from build123d import *

# Parameters (mm, degrees)
SKETCH2_W           = 635
SKETCH2_H           = 635
BOSS_EXTRUDE3_DEPTH = 4.445
SKETCH3_R           = 3.175
SKETCH3_R_2         = 3.9751
CUT_EXTRUDE1_DEPTH  = 631.349772348
SKETCH4_W           = 635
SKETCH4_H           = 635
SKETCH4_R           = 3.175
CUT_EXTRUDE2_DEPTH  = 631.349772348


with BuildPart() as part:
    # Sketch2 → Boss-Extrude3 (new body)
    with BuildSketch(Plane.XY):
        with Locations((164.767692446, -88.380463065)):
            Rectangle(SKETCH2_W, SKETCH2_H)
    extrude(amount=BOSS_EXTRUDE3_DEPTH)

    # Sketch3 → Cut-Extrude1 (cut, through all)
    with BuildSketch(Plane(origin=(0, 0, 0), x_dir=(-1, 0, 0), z_dir=(0, 0, -1))):
        with Locations((-138.143199548, 71.871365193)):
            Circle(SKETCH3_R)
        with Locations((-198.809547248, -25.000118004)):
            Circle(SKETCH3_R)
        with Locations((-122.004659563, -96.265887155)):
            Circle(SKETCH3_R)
        with Locations((-26.754659563, 23.469712845)):
            Circle(SKETCH3_R_2)
    extrude(amount=-CUT_EXTRUDE1_DEPTH, mode=Mode.SUBTRACT)

    # Sketch4 → Cut-Extrude2 (cut, through all)
    # profile 1 of 9: a face of its own
    with BuildSketch(Plane.XY.offset(4.445)):
        with Locations((164.767692446, -88.380463065)):
            Rectangle(SKETCH4_W, SKETCH4_H)
        with BuildLine():
            Line((-77.2226341, -77.634727654), (8.633248965, 17.594597704))
            ThreePointArc((8.633248965, 17.594597704), (15.63151489, 38.935098471), (38.089671454, 38.780493538))
            Line((38.089671454, 38.780493538), (119.216168571, 74.032383096))
            ThreePointArc((119.216168571, 74.032383096), (143.785411305, 90.066637834), (154.972256192, 62.944699943))
            Line((154.972256192, 62.944699943), (198.125737804, -5.962394804))
            ThreePointArc((198.125737804, -5.962394804), (212.645203515, -11.905190907), (217.780898828, -26.729371954))
            Line((217.780898828, -26.729371954), (291.816561623, -78.971587768))
            ThreePointArc((291.816561623, -78.971587768), (317.962531349, -102.027327271), (283.306875621, -105.790887155))
            Line((283.306875621, -105.790887155), (138.502443505, -105.790887155))
            ThreePointArc((138.502443505, -105.790887155), (122.004659563, -115.315887155), (105.506875621, -105.790887155))
            Line((105.506875621, -105.790887155), (-64.697556495, -105.790887155))
            ThreePointArc((-64.697556495, -105.790887155), (-98.60087325, -104.008621005), (-77.2226341, -77.634727654))
        make_face(mode=Mode.SUBTRACT)
    # profile 2 of 9: a face of its own
    with BuildSketch(Plane.XY.offset(4.445)):
        with BuildLine():
            Line((146.273652248, -86.740887155), (269.785475941, -86.740887155))
            Line((269.785475941, -86.740887155), (206.797645188, -42.294417391))
            ThreePointArc((206.797645188, -42.294417391), (200.080272342, -44.007689067), (193.194620104, -43.203828976))
            Line((193.194620104, -43.203828976), (146.273652248, -86.740887155))
        make_face()
    # profile 3 of 9: a face of its own
    with BuildSketch(Plane.XY.offset(4.445)):
        Polygon((144.946705866, 43.06176458), (140.928758156, 1.201305791), (177.638536292, -9.140258814), align=None)
    # profile 4 of 9: a face of its own
    with BuildSketch(Plane.XY.offset(4.445)):
        Polygon((179.886249099, -29.564951481), (139.079100318, -18.069110674), (133.87810257, -72.255020413), align=None)
    # profile 5 of 9: a face of its own
    with BuildSketch(Plane.XY.offset(4.445)):
        with BuildLine():
            Line((55.070704112, 25.388502171), (122.29505865, 6.450632186))
            Line((122.29505865, 6.450632186), (127.085491453, 56.359125133))
            ThreePointArc((127.085491453, 56.359125133), (126.946386449, 56.459231128), (126.808187657, 56.5605845))
            Line((126.808187657, 56.5605845), (55.070704112, 25.388502171))
        make_face()
    # profile 6 of 9: a face of its own
    with BuildSketch(Plane.XY.offset(4.445)):
        Polygon((120.445400812, -12.81978428), (52.587094953, 6.296677047), (114.776579601, -71.879651121), align=None)
    # profile 7 of 9: a face of its own
    with BuildSketch(Plane.XY.offset(4.445)):
        with BuildLine():
            Line((102.256257742, -86.740887155), (29.57120013, 4.629075933))
            ThreePointArc((29.57120013, 4.629075933), (26.167164867, 4.428774056), (22.781953227, 4.838553344))
            Line((22.781953227, 4.838553344), (-59.783303905, -86.740887155))
            Line((-59.783303905, -86.740887155), (102.256257742, -86.740887155))
        make_face()
    # profile 8 of 9: a face of its own
    with BuildSketch(Plane.XY.offset(4.445)):
        with Locations((299.804659563, -96.265887155)):
            Circle(SKETCH4_R)
    # profile 9 of 9: a face of its own
    with BuildSketch(Plane.XY.offset(4.445)):
        with Locations((-81.195340437, -96.265887155)):
            Circle(SKETCH4_R)
    extrude(amount=-CUT_EXTRUDE2_DEPTH, mode=Mode.SUBTRACT)


solid = part.part
For this review, take the finished solid that the model builds, in its own axes (mm). A direction names the side the tool comes from. Coordinates: 2 decimals unless noted, no trailing zeros. Loops run counter-clockwise (first coordinate to the right, second up) from the corner with the lowest first, then second, coordinate; pieces in that order, holes last. Notation, with made-up numbers: (-26.75, 87) - (12.25, 87) arc R31 ccw to (12.25, 115) - close; hole circle Ø2 at (-11.75, 61.25). An arc over 180 degrees is marked (long way). Return JSON: item names as keys, results as strings.
Item 1: Insertion check: pin 1 (5.5 mm diameter, centred on x = 138.14, y = 71.87, fed in from -Z); pin 2 (2 mm diameter, centred on x = 207, z = 1.5, fed in from -Y); pin 3 (2 mm diameter, centred on x = 50.5, z = 3, fed in from +Y). Each pin has a flat end and moves straight along its axis. Give the tip position at first contact, or say it passes through.
Determined:
{"pin 1": "passes through", "pin 2": "stops at y = -105.79", "pin 3": "stops at y = 44.61"}
Item 2: Mouldability with a two-part tool opening along X and no side actions: class faces 3 (the cylindrical face through (143.34, 90.2, 2.25)), 4 (the flat face through (124, -27, 0)), 5 (the cylindrical face through (122.284, -115.314, 2.254)) as pulls with the +X half, pulls with the -X half, needs draft (parallel to the pull), parting line crosses it, or undercut.
Determined:
{"face 3": "parting line crosses it", "face 4": "needs draft", "face 5": "undercut"}
Item 3: For line 1 (X direction, y = 33, z = 1.35); line 2 (Y direction, x = 177, z = 0.3); line 3 (X direction, y = -63, z = 1.8), list the stretches that pass through material, from the lowest coordinate up.
Determined:
{"line 1": "x = 10.26 to 72.59, 124.84 to 143.98, 151.25 to 173.73", "line 2": "y = -105.79 to -86.74, -58.23 to -32.24, -28.75 to -8.96, -8.12 to 27.77", "line 3": "x = -64.03 to -38.38, 83.37 to 107.71, 115.63 to 134.77, 143.85 to 171.86, 236.14 to 269.18"}
Item 4: Take a section at D-D (z = 2.9). State how many separate pieces and enclosed holes the cut face has, then the cut area to 3 significant figures.
Determined:
{"separate pieces": "1", "enclosed holes": "12", "area": "27,800 mm2"}
Item 5: For faces 1 (the flat face through (124, -27, 4.445)), 2 (the flat face through (91, 41, 2)), list the 3-axis set-ups (+Z, -Z, +X, -X, +Y, -Y) from which the entire face can be reached by the end or side of a thin tool; tool diameter is ignored.
Determined:
{"face 1": "+Z, +X, -X, +Y, -Y", "face 2": "+Z, -Z"}
Item 6: Take a section at B-B (x = 91). Give the boundary of the cut face in (y, z) (3 decimals), then the cut area to 3 significant figures.
Determined:
{"outline": "(-105.791, 0) - (-86.741, 0) - (-86.741, 4.445) - (-105.791, 4.445) - close; (-72.591, 0) - (-41.991, 0) - (-41.991, 4.445) - (-72.591, 4.445) - close; (-4.525, 0) - (15.267, 0) - (15.267, 4.445) - (-4.525, 4.445) - close; (41.001, 0) - (61.772, 0) - (61.772, 4.445) - (41.001, 4.445) - close", "area": "401 mm2"}
Item 7: Take a section at C-C (x = 211). Give the boundary of the cut face in (y, z) (3 decimals), then the cut area to 3 significant figures.
Determined:
{"outline": "(-105.791, 0) - (-86.741, 0) - (-86.741, 4.445) - (-105.791, 4.445) - close; (-45.26, 0) - (-10.361, 0) - (-10.361, 4.445) - (-45.26, 4.445) - close", "area": "240 mm2"}
Item 8: Take a section at A-A (x = -33). Give the boundary of the cut face in (y, z) (3 decimals), then the cut area to 3 significant figures.
Determined:
{"outline": "(-105.791, 0) - (-86.741, 0) - (-86.741, 4.445) - (-105.791, 4.445) - close; (-57.033, 0) - (-28.584, 0) - (-28.584, 4.445) - (-57.033, 4.445) - close", "area": "211 mm2"}
